The listing builds one solid part. Answer for the finished solid, in the listing's coordinates (mm). Coordinates: 2 decimals unless noted, no trailing zeros. Write each loop counter-clockwise with the first axis right and the second up, starting at its lowest first coordinate (ties: lowest second). Pieces come first, ordered by that corner, then holes.
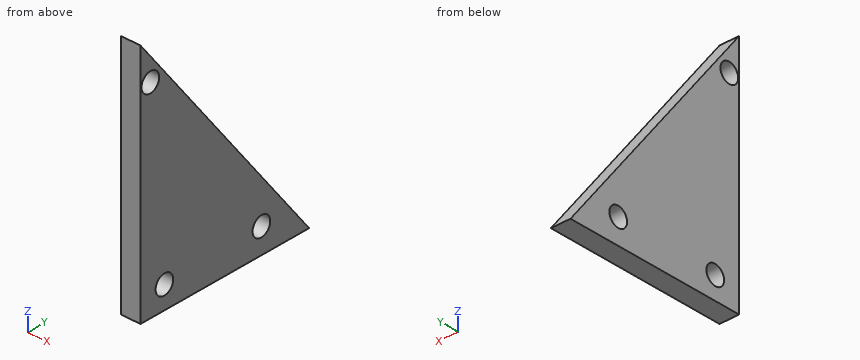
from build123d import *

# Parameters (mm, degrees)
F1_DEPTH = 5
F3_D     = 5
F5_D     = 5
F7_D     = 5


with BuildPart() as f1:
    # F0 (on Right) → F1 (new body)
    with BuildSketch(Plane.YZ):
        Polygon((24.703234, -23.224443), (-22.944346, 40.005997), (-22.944346, -22.325426), align=None)
    extrude(amount=F1_DEPTH)

    # F3 (through all)
    with Locations(Plane.YZ.offset(5)):
        with Locations((11.219002, -16.476458)):
            Hole(F3_D / 2)

    # F5 (through all)
    with Locations(Plane.YZ.offset(5)):
        with Locations((-16.186237, -16.636005)):
            Hole(F5_D / 2)

    # F7 (through all)
    with Locations(Plane.YZ.offset(5)):
        with Locations((-20.151891, 30.455533)):
            Hole(F7_D / 2)


solid = f1.part
1. Flat-ended cylindrical pins translate along their axes: P1, Ø8, axis at y = -20.15, z = 30.46, coming from the -X side; P2, Ø2, axis at y = 4, z = 7.5, coming from the +X side; P3, Ø1.5, axis at x = 3.5, y = 1.5, coming from the -Z side; P4, Ø2, axis at x = 4.5, z = 15, coming from the +Y side. Find the tip coordinate at first contact, or state that the pin passes through.
Results found:
P1: stops at x = 0
P2: passes through
P3: stops at z = -22.8
P4: stops at y = -3.35
2. Find the intervals of material crossed by L1, parallel to Y at x = 3.6, z = 30.5; L2, parallel to Y at x = 3.4, z = 31; L3, parallel to Y at x = 0.75, z = 0, in increasing order.
Results found:
L1: y = -22.94 to -22.65, -17.65 to -15.78
L2: y = -22.94 to -22.59, -17.71 to -16.16
L3: y = -22.94 to 7.2
3. Section A-A on z = 29 is taken. Give the vertices of the cut face in (x, y).
Results found:
outline: (0, -22.94) - (5, -22.94) - (5, -22.18) - (0, -22.18) - close; (0, -18.12) - (5, -18.12) - (5, -14.65) - (0, -14.65) - close
4. Section C-C on y = 7.5 is taken. Give the vertices of the cut face in (x, z) (3 decimals).
Results found:
outline: (0, -22.9) - (5, -22.9) - (5, -0.395) - (0, -0.395) - close
5. Section B-B on x = 4.2 is taken. Give the vertices of the cut face in (y, z).
Results found:
outline: (-22.94, -22.33) - (24.7, -23.22) - (-22.94, 40.01) - close; hole circle Ø5 at (-20.15, 30.46); hole circle Ø5 at (-16.19, -16.64); hole circle Ø5 at (11.22, -16.48)
6. Section D-D on z = 22.5 is taken. Give the vertices of the cut face in (x, y), then the cut area to 3 significant figures.
Results found:
outline: (0, -22.94) - (5, -22.94) - (5, -9.75) - (0, -9.75) - close
area: 66.0 mm2
